The model under review builds one solid part; all positions refer to its coordinate system, in mm. A direction names the side the tool comes from. Give positions to 0.01 mm unless a question says otherwise; leave off trailing zeros. Loops run counter-clockwise (first coordinate to the right, second up) from the corner with the lowest first, then second, coordinate; pieces in that order, holes last. Notation, with made-up numbers: M -3,12 L 47,12 A27 ccw 47,41 Z; hole C 0,73.25 d1. An arc over 180 degrees is marked long. Return JSON: item names as keys, results as strings.
```python
from build123d import *

# Parameters (mm, degrees)
BOSS_EXTRUDE1_DEPTH = 25.4
FILLET1_R           = 12.7
CUT_EXTRUDE1_DEPTH  = 94.010697189


with BuildPart() as part:
    # Sketch2 → Boss-Extrude1 (new body)
    with BuildSketch(Plane.XY):
        Polygon((0, 0), (0, 3.175), (25.4, 3.175), (85.07048142, 24.893279101), (86.156395375, 21.90975503), (25.959838164, 0), align=None)
    extrude(amount=BOSS_EXTRUDE1_DEPTH)

    # Fillet1
    fillet1_edges = [part.edges().sort_by_distance(p)[0] for p in [
        (25.4, 3.175, 12.7),
        (25.959838164, 0, 12.7),
    ]]
    fillet(fillet1_edges, radius=FILLET1_R)

    # Sketch3 → Cut-Extrude1 (cut, through all)
    with BuildSketch(Plane(origin=(1.950810242, -5.35980709, 0), x_dir=(0.9396926207859078, 0.3420201433256703, 0), z_dir=(-0.3420201433256703, 0.9396926207859079, 0))):
        Polygon((88.454106523, 0), (84.971991459, 0), (88.454106523, -3.482115064), align=None)
        Polygon((88.454106523, -25.4), (88.454106523, -21.917884936), (84.971991459, -25.4), align=None)
    extrude(amount=-CUT_EXTRUDE1_DEPTH, mode=Mode.SUBTRACT)


solid = part.part
```
1) The part is to be moulded in two halves that separate along X. For faces 1 (the face through (85.606, 23.422, 12.571)), 2 (the face through (25.335, 3.363, 12.878)), 3 (the face through (42, 8, 25.4)), say which applies: released by +X, released by -X, zero draft, split by the parting line, or undercut.
From the geometry:
{"face 1": "released by +X", "face 2": "released by -X", "face 3": "zero draft"}
2) Insertion check: pin 1 (1.5 mm diameter, centred on x = 62, z = 5, fed in from +Y); pin 2 (7 mm diameter, centred on x = 9.5, z = 11.5, fed in from +Y) (3 decimals); pin 3 (10 mm diameter, centred on x = 26.5, z = 10.5, fed in from +Y). Each pin has a flat end and moves straight along its axis. Give the tip position at first contact, or say it passes through.
From the geometry:
{"pin 1": "y = 16.77", "pin 2": "y = 3.175", "pin 3": "y = 5.4"}
3) Consider section C-C on y = 17.75. Write out the cut boundary in (x, z).
From the geometry:
{"outline": "M 65.44,0 L 74.73,0 L 74.73,25.4 L 65.44,25.4 Z"}
4) Tool access review of faces 4 (the face through (11, 3.175, 13)), 5 (the face through (12, 0, 13)): name each direction out of +Z, -Z, +X, -X, +Y, -Y from which nothing blocks a thin tool from reaching the whole face with its end or side.
From the geometry:
{"face 4": "+Z, -Z, -X, +Y", "face 5": "+Z, -Z, +X, -X, -Y"}
5) Consider section B-B on x = 12. Write out the cut boundary in (y, z) (3 decimals).
From the geometry:
{"outline": "M 0,0 L 3.175,0 L 3.175,25.4 L 0,25.4 Z"}
6) Consider section A-A on z = 16.5. Write out the cut boundary in (x, y) (3 decimals).
From the geometry:
{"outline": "M 0,0 L 23.72,0 A12.7 ccw 28.064,0.766 L 86.156,21.91 L 85.07,24.893 L 27.504,3.941 A12.7 cw 23.161,3.175 L 0,3.175 Z"}
7) Wall thickness on L1, parallel to Y at x = 18, z = 19.5 (3 decimals); L2, parallel to Y at x = 51.5, z = 23: over which ranges is each line inside the solid? List them lowest first. Write a range as from..to.
From the geometry:
{"L1": "0..3.175", "L2": "9.3..12.67"}
